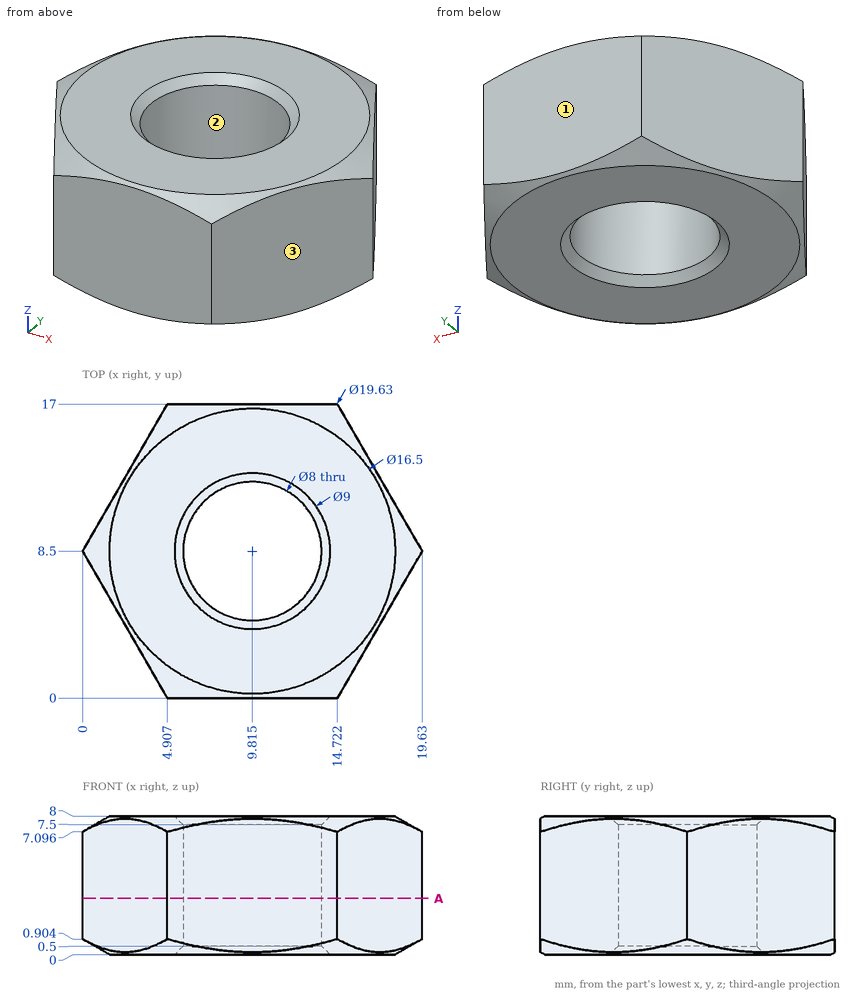
Design review of the part shown in the three views and the two pictorial views. Dimensions are in mm from the part's minimum x, y and z. Round coordinates to 2 decimals unless told otherwise and drop trailing zeros. Loops run counter-clockwise (first coordinate to the right, second up) from the corner with the lowest first, then second, coordinate; pieces in that order, holes last.
1) Consider section A-A on z = 3.25. State the section outline as (x, y) points (1 decimal).
Values follow:
outline: (0, 8.5) - (4.9, 0) - (14.7, 0) - (19.6, 8.5) - (14.7, 17) - (4.9, 17) - close; hole circle Ø8 at (9.8, 8.5)
2) Clearance check with flat-ended pins moving along their axes: P1, Ø3, axis at x = 12, y = 12, coming from the -Z side; P2, Ø6.5, axis at x = 9.81, y = 8.5, coming from the -Z side; P3, Ø1, axis at y = 14, z = 2, coming from the -X side; P4, Ø1, axis at x = 8, y = 12, coming from the +Z side. State where each tip first meets the part, or that it passes through.
Values follow:
P1: stops at z = 0
P2: passes through
P3: stops at x = 2.89
P4: stops at z = 7.94
3) The part is to be moulded in two halves that separate along X. For the marked faces 1, 2 and 3, say which applies: pulls with the +X half, pulls with the -X half, needs draft (parallel to the pull), parting line crosses it, or undercut.
Values follow:
face 1: needs draft
face 2: undercut
face 3: pulls with the +X half
4) Wall thickness on line 1 along Y through (x, z) = (13.25, 1); line 2 along Y through (x, z) = (11.75, 1.5); line 3 along X through (y, z) = (8.25, 3.5) (1 decimal): over which ranges is each line inside the solid? List them lowest first.
Values follow:
line 1: y = 0 to 6.45, 10.55 to 17
line 2: y = 0 to 5, 12 to 17
line 3: x = 0.1 to 5.8, 13.8 to 19.5
